Drawing for the job (mm, zero at the part's lowest x, y, z). Round coordinates to 2 decimals unless told otherwise and drop trailing zeros. Loops run counter-clockwise (first coordinate to the right, second up) from the corner with the lowest first, then second, coordinate; pieces in that order, holes last.
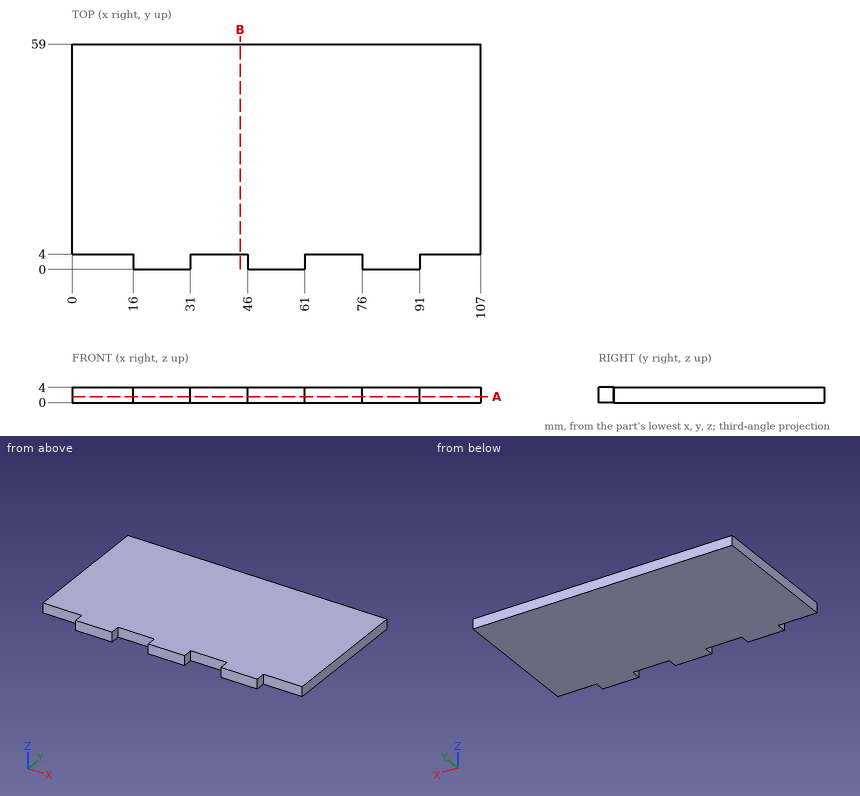
Q1. Probe line 1 (Y direction, x = 14, z = 1.45). List the from-to ranges inside material, lowest first.
Q2. Slice it at A-A on z = 1.6. Give the cut face in (x, y).
Q3. Flat gauge pins, fed straight in: P1, Ø2, axis at y = 2.5, z = 2.5, coming from the +X side; P2, Ø2, axis at x = 42, z = 1.5, coming from the -Y side; P3, Ø1.2, axis at y = 2.5, z = 2.5, coming from the -X side. Where does each tip first touch, or does it go through?
Q4. Slice it at B-B on x = 44. Give the cut face in (y, z), plus the area to 3 significant figures.
Reply:
1. line 1: y = 4 to 59
2. outline: (0, 4) - (16, 4) - (16, 0) - (31, 0) - (31, 4) - (46, 4) - (46, 0) - (61, 0) - (61, 4) - (76, 4) - (76, 0) - (91, 0) - (91, 4) - (107, 4) - (107, 59) - (0, 59) - close
3. P1: stops at x = 91
3. P2: stops at y = 4
3. P3: stops at x = 16
4. outline: (4, 0) - (59, 0) - (59, 4) - (4, 4) - close
4. area: 220 mm2
